The listing builds one solid part. Answer for the finished solid, in the listing's coordinates (mm). A direction names the side the tool comes from. Coordinates: 2 decimals unless noted, no trailing zeros. Write each loop counter-clockwise with the first axis right and the second up, starting at its lowest first coordinate (ties: lowest second). Pieces come first, ordered by that corner, then holes.
(1) Which of the six approach directions +Z, -Z, +X, -X, +Y, -Y give full straight-line access (tool end or side, diameter ignored) to faces 1 (the flat face through (95, -36, -33.5)), 2 (the flat face through (89, -74, -30.2)), 3 (the flat face through (89, 37, -30.2)), 4 (the flat face through (83, -36, -33.5))?
(2) Straight lines are drawn through the part: line 1 (Y direction, x = 82.96, z = -28.55); line 2 (X direction, y = -32.25, z = -28.35); line 3 (Z direction, x = 87.5, y = 75). For each, find the intervals that lie inside material, in ascending order.
(3) The part is cut by section B-B on y = 71.5. Determine the outline of the cut face in (x, z), plus the area to 3 significant figures.
(4) The part is cut by section A-A on x = 89.75. Determine the outline of the cut face in (y, z), plus the area to 3 significant figures.
(5) Given P1, Ø1.9, axis at x = 83.5, y = -32.5, coming from the +Z side; P2, Ø2, axis at x = 82.96, y = -40.25, coming from the -Z side; P3, Ø1, axis at y = 46.5, z = -30.5, coming from the +X side; P4, Ø1.5, axis at x = 86, y = -77.5, coming from the +Z side, each flat-ended and moving along its own axis, determine where each tip first touches the part or whether it passes through.
from build123d import *

# Parameters (mm, degrees)
SKETCH022_W     = 7
SKETCH022_H     = 4.8
PAD008_DEPTH    = 200
SKETCH023_W     = 17
SKETCH023_H     = 22.5
PAD009_DEPTH    = 6.5
SKETCH025_W     = 17
SKETCH025_H     = 4.5
POCKET014_DEPTH = 0.1
SKETCH024_R     = 1.2
POCKET015_DEPTH = 2.5


with BuildPart() as part:
    # Sketch022 → Pad008 (new body)
    with BuildSketch(Plane.XZ):
        with Locations((3.5, 2.4)):
            Rectangle(SKETCH022_W, SKETCH022_H)
    extrude(amount=-PAD008_DEPTH)

    # Sketch023 (on Face1 of Pad008) → Pad009 (join)
    with BuildSketch(Plane(origin=(0, 0, 1.5), x_dir=(-1, 0, 0), z_dir=(0, 0, 1))):
        with Locations((-3.5, -63.75)):
            Rectangle(SKETCH023_W, SKETCH023_H)
    extrude(amount=PAD009_DEPTH)

    # Sketch025 (on Face13 of Pad009) → Pocket014 (cut)
    with BuildSketch(Plane(origin=(0, 0, 8), x_dir=(-1, 0, 0), z_dir=(0, 0, 1))):
        with Locations((-3.5, -54.75)):
            Rectangle(SKETCH025_W, SKETCH025_H)
        with Locations((-3.5, -72.75)):
            Rectangle(SKETCH025_W, SKETCH025_H)
    extrude(amount=-POCKET014_DEPTH, mode=Mode.SUBTRACT)

    # Sketch024 (on Face17 of Pocket014) → Pocket015 (cut)
    with BuildSketch(Plane(origin=(0, 0, 8), x_dir=(-1, 0, 0), z_dir=(0, 0, 1))):
        with Locations((-9.5, -59.75)):
            Circle(SKETCH024_R)
        with Locations((2.5, -59.75)):
            Circle(SKETCH024_R)
        with Locations((2.5, -67.75)):
            Circle(SKETCH024_R)
        with Locations((-9.5, -67.75)):
            Circle(SKETCH024_R)
    extrude(amount=-POCKET015_DEPTH, mode=Mode.SUBTRACT)


with BuildPart() as part_1:
    # Body005 placement: moved
    add(part.part.moved(Location((85.46, -100, -35))))


solid = part_1.part
Model answer:
1. face 1: -Z, +X, +Y, -Y
1. face 2: +Z, +X, -X, -Y
1. face 3: +Z, +X, -X, +Y
1. face 4: -Z, -X, +Y, -Y
2. line 1: y = -47.5 to -41.45, -39.05 to -33.45, -31.05 to -25
2. line 2: x = 80.46 to 81.76, 84.16 to 93.76, 96.16 to 97.46
2. line 3: z = -35 to -30.2
3. outline: (85.46, -35) - (92.46, -35) - (92.46, -30.2) - (85.46, -30.2) - close
3. area: 33.6 mm2
4. outline: (-100, -35) - (100, -35) - (100, -30.2) - (-25, -30.2) - (-25, -27.1) - (-29.5, -27.1) - (-29.5, -27) - (-43, -27) - (-43, -27.1) - (-47.5, -27.1) - (-47.5, -30.2) - (-100, -30.2) - close
4. area: 1,030 mm2
5. P1: stops at z = -27
5. P2: stops at z = -33.5
5. P3: stops at x = 92.46
5. P4: stops at z = -30.2
